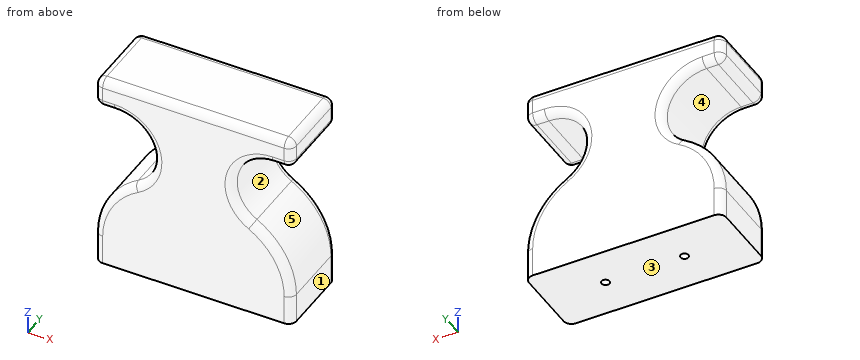
from build123d import *

# Parameters (mm, degrees)
PAD001_DEPTH    = 10
FILLET_R        = 2
SKETCH003_R     = 1
POCKET001_DEPTH = 20


with BuildPart() as part:
    # Sketch002 → Pad001 (new body, symmetric)
    with BuildSketch(Plane.XZ):
        with BuildLine():
            Line((-25, 0), (-25, 7.5))
            ThreePointArc((-15, 24.820508), (-22.320508, 17.5), (-25, 7.5))
            ThreePointArc((-15, 24.820508), (-10.340742, 36.068953), (-20, 43.480762))
            Line((-20, 43.480762), (-25, 43.480762))
            Line((-25, 43.480762), (-25, 50.980762))
            Line((-25, 50.980762), (0, 50.980762))
            Line((0, 50.980762), (0, 0))
            Line((0, 0), (-25, 0))
        make_face()
    pad001 = extrude(amount=PAD001_DEPTH, both=True)

    # Mirrored: Pad001 across Sketch002 V_Axis
    add(pad001.mirror(Plane(origin=(0, 0, 0), x_dir=(0, -1, 0), z_dir=(1, 0, 0))))

    # Fillet
    fillet_edges = [part.edges().sort_by_distance(p)[0] for p in [
        (25, 0, 43.480762),
        (25, 0, 50.980762),
        (25, 10, 47.230762),
        (25, -10, 47.230762),
        (-25, 0, 43.480762),
        (-25, 0, 50.980762),
        (-25, 10, 47.230762),
        (-25, -10, 47.230762),
        (0, -10, 50.980762),
        (0, 10, 50.980762),
        (22.5, -10, 43.480762),
        (10.340742, -10, 36.068953),
        (22.320508, -10, 17.5),
        (25, -10, 3.75),
        (25, 10, 3.75),
        (22.320508, 10, 17.5),
        (10.340742, 10, 36.068953),
        (22.5, 10, 43.480762),
        (-25, 10, 3.75),
        (-22.320508, 10, 17.5),
        (-10.340742, 10, 36.068953),
        (-22.5, 10, 43.480762),
        (-22.5, -10, 43.480762),
        (-10.340742, -10, 36.068953),
        (-22.320508, -10, 17.5),
        (-25, -10, 3.75),
    ]]
    fillet(fillet_edges, radius=FILLET_R)

    # Sketch003 (on Face2 of Fillet) → Pocket001 (cut)
    with BuildSketch(Plane(origin=(0, 0, 0), x_dir=(1, 0, 0), z_dir=(0, 0, -1))):
        with Locations((-10, 0)):
            Circle(SKETCH003_R)
        with Locations((10, 0)):
            Circle(SKETCH003_R)
    extrude(amount=-POCKET001_DEPTH, mode=Mode.SUBTRACT)


solid = part.part
Here's how the part is built. I have some questions about the finished solid (model axes, mm). Face numbers are marked on the shaded views. A direction names the side the tool comes from. Round coordinates to 2 decimals unless told otherwise and drop trailing zeros. Write each loop counter-clockwise with the first axis right and the second up, starting at its lowest first coordinate (ties: lowest second). Pieces come first, ordered by that corner, then holes. Notation, with made-up numbers: (54, -19) -> (77, -19) arc R26 cw to (77, -5) -> close; hole circle Ø7 at (-40, 76). An arc over 180 degrees is marked (long way). One line per item, written item: value.
1) For the marked faces 4 and 5, which set-ups out of +Z, -Z, +X, -X, +Y, -Y let a thin tool reach every point of the face, with its end or its side?
Filled sheet:
face 4: -X, +Y, -Y
face 5: +X, +Y, -Y
2) Suppose I cut it at C-C on y = -4.25. List the corners of the cut face in (x, z) for me.
Filled sheet:
outline: (-25, 0) -> (25, 0) -> (25, 7.5) arc R20 ccw to (15, 24.82) arc R10 cw to (20, 43.48) -> (23, 43.48) arc R2 ccw to (25, 45.48) -> (25, 48.98) arc R2 ccw to (23, 50.98) -> (-23, 50.98) arc R2 ccw to (-25, 48.98) -> (-25, 45.48) arc R2 ccw to (-23, 43.48) -> (-20, 43.48) arc R10 cw to (-15, 24.82) arc R20 ccw to (-25, 7.5) -> close
3) If I drill on line 1 (X direction, y = 0, z = 7); line 2 (Y direction, x = 10, z = 15); line 3 (X direction, y = 0, z = 15.5), over which ranges is the centre line in solid material (lowest first)? Write a range as [from, to].
Filled sheet:
line 1: x = [-25, -11], [-9, 9], [11, 25]
line 2: y = [-10, -1], [1, 10]
line 3: x = [-23.33, -11], [-9, 9], [11, 23.33]
4) We'd pull the mould along Z, two halves only. Please class the marked faces 1, 2 and 3: released by +Z, released by -Z, zero draft, split by the parting line, or undercut.
Filled sheet:
face 1: zero draft
face 2: undercut
face 3: released by -Z
5) I'm going to push flat-ended pins straight in: pin 1 Ø1 at (y, z) = (4.5, 24) entering from -X; pin 2 Ø2 at (x, z) = (14.5, 41) entering from +Y; pin 3 Ø6 at (y, z) = (2, 18) entering from +X. Where does each tip first touch, or does it pass through?
Filled sheet:
pin 1: stops at x = -17
pin 2: stops at y = 9.08
pin 3: stops at x = 23.54
6) Suppose I cut it at B-B on z = 17.5. Give the number of separate pieces and of enclosed holes in the cut face, plus the area to 3 significant figures.
Filled sheet:
separate pieces: 1
enclosed holes: 2
area: 883 mm2
7) Suppose I cut it at A-A on y = 0. List the corners of the cut face in (x, z) for me.
Filled sheet:
outline: (-25, 0) -> (-11, 0) -> (-11, 20) -> (-9, 20) -> (-9, 0) -> (9, 0) -> (9, 20) -> (11, 20) -> (11, 0) -> (25, 0) -> (25, 7.5) arc R20 ccw to (15, 24.82) arc R10 cw to (20, 43.48) -> (23, 43.48) arc R2 ccw to (25, 45.48) -> (25, 48.98) arc R2 ccw to (23, 50.98) -> (-23, 50.98) arc R2 ccw to (-25, 48.98) -> (-25, 45.48) arc R2 ccw to (-23, 43.48) -> (-20, 43.48) arc R10 cw to (-15, 24.82) arc R20 ccw to (-25, 7.5) -> close
